from build123d import *

# Parameters (mm, degrees)
BOSS_EXTRUDE1_DEPTH = 800
SKETCH2_R           = 1.5
CUT_EXTRUDE1_DEPTH  = 205
SKETCH3_R           = 1.5
CUT_EXTRUDE2_DEPTH  = 25


with BuildPart() as part:
    # Sketch1 → Boss-Extrude1 (new body)
    with BuildSketch(Plane(origin=(0, 0, 0), x_dir=(0, 0, -1), z_dir=(1, 0, 0))):
        with BuildLine():
            Line((-9.5, -10), (9.5, -10))
            ThreePointArc((9.5, -10), (9.853553391, -9.853553391), (10, -9.5))
            Line((10, -9.5), (10, 9.5))
            ThreePointArc((10, 9.5), (9.853553391, 9.853553391), (9.5, 10))
            Line((9.5, 10), (-9.5, 10))
            ThreePointArc((-9.5, 10), (-9.853553391, 9.853553391), (-10, 9.5))
            Line((-10, 9.5), (-10, -9.5))
            ThreePointArc((-10, -9.5), (-9.853553391, -9.853553391), (-9.5, -10))
        make_face()
        with BuildLine():
            Line((-8, -9), (8, -9))
            ThreePointArc((8, -9), (8.707106781, -8.707106781), (9, -8))
            Line((9, -8), (9, 8))
            ThreePointArc((9, 8), (8.707106781, 8.707106781), (8, 9))
            Line((8, 9), (-8, 9))
            ThreePointArc((-8, 9), (-8.707106781, 8.707106781), (-9, 8))
            Line((-9, 8), (-9, -8))
            ThreePointArc((-9, -8), (-8.707106781, -8.707106781), (-8, -9))
        make_face(mode=Mode.SUBTRACT)
    extrude(amount=BOSS_EXTRUDE1_DEPTH)

    # Sketch2 → Cut-Extrude1 (cut)
    with BuildSketch(Plane.XY.offset(10)):
        with Locations((792, 0)):
            Circle(SKETCH2_R)
        with Locations((772, 0)):
            Circle(SKETCH2_R)
    extrude(amount=-CUT_EXTRUDE1_DEPTH, mode=Mode.SUBTRACT)

    # Sketch3 → Cut-Extrude2 (cut)
    with BuildSketch(Plane.XY.offset(10)):
        with Locations((8, 0)):
            Circle(SKETCH3_R)
        with Locations((28, 0)):
            Circle(SKETCH3_R)
    extrude(amount=-CUT_EXTRUDE2_DEPTH, mode=Mode.SUBTRACT)


solid = part.part
Geometry: final body of the model. Coordinates: model frame, mm. A direction names the side the tool comes from. Give positions to 0.01 mm unless a question says otherwise; leave off trailing zeros. Write each loop counter-clockwise with the first axis right and the second up, starting at its lowest first coordinate (ties: lowest second). Pieces come first, ordered by that corner, then holes. Notation, with made-up numbers: (68, 16) - (94, 16) arc R23 ccw to (94, 29) - close; hole circle Ø10 at (-31.5, -31.5). An arc over 180 degrees is marked (long way). Return JSON: item names as keys, results as strings. Group by question number.
1) First-contact query: P1, Ø3.5, axis at x = 28, y = 0, coming from the +Z side. Flat tip, straight axial feed; report the tip coordinate or a pass-through.
2) Section A-A on z = 1.5. Return the cut outline in (x, y), plus the area to 3 significant figures.
3) Mould query, pull axis Z, two halves, no side actions, for faces 1 (the flat face through (394, 9, 0)), 2 (the flat face through (0, 9.7, 0)), 3 (the flat face through (394, 0, 10)). Classes: released by +Z, released by -Z, zero draft, split by the parting line, or undercut.
4) Line query: line 1 (Y direction, x = 772, z = -9.45); line 2 (Z direction, x = 156.5, y = 3.5). Output: solid intervals per line, ascending.
5) Section B-B on x = 238. Return the cut outline in (y, z), plus the area to 3 significant figures.
6) Set-up query: faces 4 (the flat face through (394, 0, -10)), 5 (the flat face through (394, -9, 0)). Return all of +Z, -Z, +X, -X, +Y, -Y with unobstructed straight access to the full face (end or side cutting, diameter ignored); none if empty.
Filled in:
{
 "1": {"P1": "stops at z = 10"},
 "2": {"outline": "(0, -10) - (800, -10) - (800, -9) - (0, -9) - close; (0, 9) - (800, 9) - (800, 10) - (0, 10) - close", "area": "1,600 mm^2"},
 "3": {"face 1": "undercut", "face 2": "zero draft", "face 3": "released by +Z"},
 "4": {"line 1": "y = -10 to -1.5, 1.5 to 10", "line 2": "z = -10 to -9, 9 to 10"},
 "5": {"outline": "(-10, -9.5) arc R0.5 ccw to (-9.5, -10) - (9.5, -10) arc R0.5 ccw to (10, -9.5) - (10, 9.5) arc R0.5 ccw to (9.5, 10) - (-9.5, 10) arc R0.5 ccw to (-10, 9.5) - close; hole (-9, -8) arc R1 ccw to (-8, -9) - (8, -9) arc R1 ccw to (9, -8) - (9, 8) arc R1 ccw to (8, 9) - (-8, 9) arc R1 ccw to (-9, 8) - close", "area": "76.6 mm^2"},
 "6": {"face 4": "-Z, +X, -X, +Y, -Y", "face 5": "+X, -X"}
}
